Build history of the part. All positions in model axes, mm. A direction names the side the tool comes from. Coordinates: 2 decimals unless noted, no trailing zeros. Loops run counter-clockwise (first coordinate to the right, second up) from the corner with the lowest first, then second, coordinate; pieces in that order, holes last.
Item 1: 3-axis set-ups, long thin cutter, end or side, ignore diameter. For faces 4 (the face through (0, 50, 0)), 5 (the face through (0, 49, -2.632)): which of +Z, -Z, +X, -X, +Y, -Y reach the whole face in a straight line?
Item 2: Mould opens along Z. For faces 1 (the face through (0, 0, 0)), 2 (the face through (-1.08, 24.65, 4.88)), 3 (the face through (-0.9, 48.52, -1.74)) say: released by +Z, released by -Z, zero draft, split by the parting line, or undercut.
Item 3: Cut at C-C (z = 3.5). List the corners of the cut face in (x, y), and give its area (3 significant figures).
Item 4: Cut at B-B (y = 30.5). List the corners of the cut face in (x, z), and give its area (3 significant figures).
Item 5: Drill centre lines: line 1 along Z through (x, y) = (-0.25, 23.5); line 2 along X through (y, z) = (36, 4.5); line 3 along X through (y, z) = (41.5, 4). Where is each one in solid material? Low to high.
Item 6: Cut at A-A (x = -4). List the corners of the cut face in (y, z), and give its area (3 significant figures).
from build123d import *

# Parameters (mm, degrees)
SKETCH1_R           = 5
BOSS_EXTRUDE1_DEPTH = 50
CUT_EXTRUDE1_DEPTH  = 3


with BuildPart() as part:
    # Sketch1 → Boss-Extrude1 (new body)
    with BuildSketch(Plane(origin=(0, 0, 0), x_dir=(1, 0, 0), z_dir=(0, 1, 0))):
        Circle(SKETCH1_R)
    extrude(amount=BOSS_EXTRUDE1_DEPTH)

    # Sketch2 → Cut-Extrude1 (cut)
    with BuildSketch(Plane(origin=(0, 50, 0), x_dir=(1, 0, 0), z_dir=(0, 1, 0))):
        with BuildLine():
            Line((0.718635203, 2.631935528), (0.718635203, 2.272961169))
            Line((0.718635203, 2.272961169), (-0.471869605, 2.272961169))
            Line((-0.471869605, 2.272961169), (-0.660471368, 1.352388253))
            add(Edge.make_bspline(
                [(-0.660471368, 1.352388253), (-0.623415494, 1.362618525), (-0.551625598, 1.382438058), (-0.445665737, 1.404443829), (-0.345073533, 1.417709273), (-0.279798163, 1.419520583), (-0.248211753, 1.420397067)],
                knots=[0, 0, 0, 0, 0.000115302, 0.000223379, 0.000324431, 0.000419176, 0.000419176, 0.000419176, 0.000419176], degree=3))
            add(Edge.make_bspline(
                [(-0.248211753, 1.420397067), (-0.209128013, 1.419551131), (-0.132279616, 1.41788781), (-0.019840669, 1.401915961), (0.087492225, 1.376776046), (0.189494595, 1.341655524), (0.286355146, 1.296745791), (0.377182707, 1.240645851), (0.46334062, 1.17511252), (0.543283214, 1.099767508), (0.615807522, 1.016845891), (0.679573512, 0.92768802), (0.733736102, 0.833160358), (0.777296857, 0.732359749), (0.812081191, 0.626400596), (0.835233186, 0.514168013), (0.850649895, 0.396719893), (0.852372281, 0.316415323), (0.853250587, 0.275465176)],
                knots=[0, 0, 0, 0, 0.00011719, 0.000230425, 0.000339944, 0.000447481, 0.000553499, 0.000659556, 0.000767111, 0.000877722, 0.000988528, 0.001097091, 0.001206056, 0.001314692, 0.001425996, 0.001539995, 0.001658004, 0.001780798, 0.001780798, 0.001780798, 0.001780798], degree=3))
            add(Edge.make_bspline(
                [(0.853250587, 0.275465176), (0.852585512, 0.246942956), (0.851264349, 0.190283968), (0.844545762, 0.106139767), (0.831610046, 0.023776934), (0.814242321, -0.056815458), (0.791699904, -0.13548483), (0.76441085, -0.212456358), (0.731014822, -0.287250965), (0.694383447, -0.36057636), (0.653136969, -0.430774867), (0.607358461, -0.496423853), (0.55899297, -0.558508135), (0.506951585, -0.616361868), (0.45075059, -0.669604886), (0.391070623, -0.718553167), (0.328387904, -0.764034497), (0.261732661, -0.804202693), (0.192590179, -0.841165649), (0.119961961, -0.871489186), (0.045501261, -0.898599714), (-0.031863615, -0.920209242), (-0.111957427, -0.937141796), (-0.194912203, -0.948642397), (-0.280292873, -0.957018834), (-0.338167885, -0.957543191), (-0.367402458, -0.957808061)],
                knots=[0, 0, 0, 0, 8.5583e-05, 0.000170009, 0.000253005, 0.000335518, 0.000417186, 0.000498352, 0.000580291, 0.000662755, 0.000744161, 0.000824288, 0.000902692, 0.000980133, 0.001057498, 0.001134702, 0.00121156, 0.001289599, 0.001368002, 0.001446531, 0.001525481, 0.001605609, 0.001687289, 0.001770875, 0.001856759, 0.001944425, 0.001944425, 0.001944425, 0.001944425], degree=3))
            add(Edge.make_bspline(
                [(-0.367402458, -0.957808061), (-0.402276638, -0.957117223), (-0.470887469, -0.955758081), (-0.571408036, -0.941539596), (-0.668122642, -0.92117568), (-0.760252743, -0.89053941), (-0.848624007, -0.852152115), (-0.932046724, -0.803635944), (-1.012652501, -0.74865684), (-1.087164537, -0.683776487), (-1.156320651, -0.612860805), (-1.21822716, -0.535903164), (-1.273360736, -0.454173722), (-1.320838483, -0.367275567), (-1.361336505, -0.275437037), (-1.393151493, -0.178314036), (-1.418829848, -0.076414032), (-1.429693268, -0.006260521), (-1.435210951, 0.029371426)],
                knots=[0, 0, 0, 0, 0.000104552, 0.000205693, 0.000304023, 0.000400691, 0.00049644, 0.000592535, 0.000689779, 0.000788716, 0.000888377, 0.000986596, 0.001084603, 0.001183757, 0.001283279, 0.001385267, 0.001490017, 0.001598135, 0.001598135, 0.001598135, 0.001598135], degree=3))
            Line((-1.435210951, 0.029371426), (-1.121108387, 0.029371426))
            add(Edge.make_bspline(
                [(-1.121108387, 0.029371426), (-1.11337983, -0.004005027), (-1.098525113, -0.068156421), (-1.065919365, -0.158287763), (-1.026053489, -0.238606986), (-0.978649141, -0.31017657), (-0.92209911, -0.372585567), (-0.857569681, -0.428202629), (-0.785221958, -0.478377758), (-0.704828729, -0.520200525), (-0.620015649, -0.555869279), (-0.531248439, -0.579620974), (-0.440944093, -0.596321867), (-0.379865723, -0.597993627), (-0.349173291, -0.598833702)],
                knots=[0, 0, 0, 0, 0.000102709, 0.000197412, 0.000286774, 0.000371169, 0.000454082, 0.000538572, 0.000626283, 0.000717552, 0.000809994, 0.00090168, 0.00099274, 0.001084718, 0.001084718, 0.001084718, 0.001084718], degree=3))
            add(Edge.make_bspline(
                [(-0.349173291, -0.598833702), (-0.319214847, -0.598012924), (-0.260226424, -0.596396806), (-0.173415038, -0.583957794), (-0.089602164, -0.564800223), (-0.009614807, -0.536130368), (0.067946733, -0.501285649), (0.141120503, -0.456570573), (0.21202338, -0.405110555), (0.278451514, -0.346153925), (0.339290963, -0.28118423), (0.393047084, -0.211706837), (0.437823998, -0.13758999), (0.475558107, -0.060116837), (0.504211405, 0.02156172), (0.524652387, 0.107062895), (0.536655445, 0.196597875), (0.538306625, 0.257667185), (0.539148023, 0.28878649)],
                knots=[0, 0, 0, 0, 8.9842e-05, 0.0001769, 0.000262612, 0.000347317, 0.000431396, 0.000517249, 0.000604055, 0.000693954, 0.000783242, 0.000870748, 0.000956963, 0.001042571, 0.001128832, 0.00121607, 0.001305907, 0.001399251, 0.001399251, 0.001399251, 0.001399251], degree=3))
            add(Edge.make_bspline(
                [(0.539148023, 0.28878649), (0.538489544, 0.316862242), (0.537200664, 0.371816531), (0.526670093, 0.452215737), (0.508353121, 0.528288779), (0.482929241, 0.600403013), (0.450649733, 0.668626456), (0.411203421, 0.733029516), (0.363850023, 0.792763349), (0.309758135, 0.847855903), (0.250500094, 0.898700778), (0.185056351, 0.942044864), (0.114796424, 0.978508782), (0.040566825, 1.00997678), (-0.039398074, 1.032577525), (-0.123514706, 1.049545411), (-0.212691414, 1.059360774), (-0.273662102, 1.060722662), (-0.305002618, 1.061422708)],
                knots=[0, 0, 0, 0, 8.4208e-05, 0.000164824, 0.000242709, 0.000318547, 0.000393815, 0.000468731, 0.000544614, 0.00062196, 0.000700062, 0.000778428, 0.000856831, 0.000937299, 0.001019835, 0.001105635, 0.00119452, 0.001288536, 0.001288536, 0.001288536, 0.001288536], degree=3))
            add(Edge.make_bspline(
                [(-0.305002618, 1.061422708), (-0.332131547, 1.060842117), (-0.388145902, 1.059643343), (-0.474068729, 1.050816846), (-0.564360452, 1.036577552), (-0.658674947, 1.016991305), (-0.757295455, 0.991360228), (-0.860013856, 0.960645727), (-0.967046123, 0.923923728), (-1.039163847, 0.896191515), (-1.076236592, 0.881935528)],
                knots=[0, 0, 0, 0, 8.1378e-05, 0.000168026, 0.000258858, 0.000355524, 0.000456875, 0.000564457, 0.000677092, 0.000796243, 0.000796243, 0.000796243, 0.000796243], degree=3))
            Line((-1.076236592, 0.881935528), (-0.717262233, 2.631935528))
            Line((-0.717262233, 2.631935528), (0.718635203, 2.631935528))
        make_face()
    extrude(amount=-CUT_EXTRUDE1_DEPTH, mode=Mode.SUBTRACT)


solid = part.part
Filled sheet:
1. face 4: +Z, -Z, +X, -X, +Y
1. face 5: +Y
2. face 1: zero draft
2. face 2: split by the parting line
2. face 3: undercut
3. outline: (-3.57, 0) - (3.57, 0) - (3.57, 50) - (-3.57, 50) - close
3. area: 357 mm2
4. outline: circle Ø10 at (0, 0)
4. area: 78.5 mm2
5. line 1: z = -4.99 to 4.99
5. line 2: x = -2.18 to 2.18
5. line 3: x = -3 to 3
6. outline: (0, -3) - (50, -3) - (50, 3) - (0, 3) - close
6. area: 300 mm2
